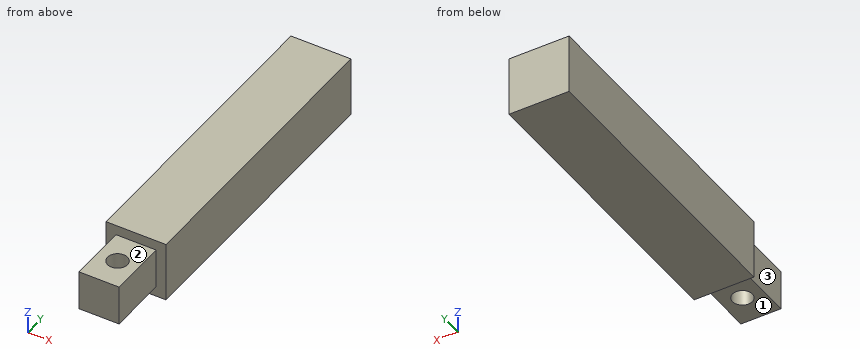
Autodesk Inventor part; units mm, degrees
ref_plane "YZ Plane" through (0, 0, 0) normal (1, 0, 0) x (0, 1, 0)
ref_plane "XZ Plane" through (0, 0, 0) normal (0, 1, 0) x (-1, 0, 0)
ref_plane "XY Plane" through (0, 0, 0) normal (0, 0, 1) x (1, 0, 0)
sketch "Sketch1" plane through (0, 0, 0) normal (0, 1, 0) x (-1, 0, 0)
  line L0 (0, 0) -> (-10, 0)
  line L1 (-10, 0) -> (-10, -10)
  line L2 (-10, -10) -> (0, -10)
  line L3 (0, -10) -> (0, 0)
  dimension "d0" = 10
  dimension "d1" = 10
extrude "Extrusion1" add sketch "Sketch1" along normal blind 15
sketch "Sketch2" plane through (0, 15, 0) normal (0, 1, 0) x (1, 0, 0)
  line L0 (12.5, -2.5) -> (-2.5, -2.5)
  line L1 (-2.5, -2.5) -> (-2.5, 12.5)
  line L2 (-2.5, 12.5) -> (12.5, 12.5)
  line L3 (12.5, 12.5) -> (12.5, -2.5)
  line L4 (12.5, -2.5) -> (-2.5, 12.5) construction
  line L5 (-2.5, -2.5) -> (12.5, 12.5) construction
  point P0 (0, 0)
  point P1 (5, 5)
  dimension "d4" = 15
  dimension "d5" = 15
extrude "Extrusion2" add sketch "Sketch2" along normal blind 75
sketch "Sketch3" plane through (0, 0, 0) normal (0, 0, 1) x (1, 0, 0)
  line L0 (0, 0) -> (0, 15)
  line L1 (0, 7.5) -> (10, 7.5)
  line L2 (10, 0) -> (10, 15)
  line L3 (-2.5, 15) -> (12.5, 15)
  line L4 (5, 15) -> (5, 0)
  line L5 (0, 0) -> (10, 0)
  point P0 (5, 7.5)
hole "Hole1" at (5, 7.5, 0) direction (0, 0, -1) diameter 5 end through all
properties part number "Pendulum"
Check sheet for the modelled part. Datum: model origin and axes. Units: mm. Face numbers are marked on the shaded views. A direction names the side the tool comes from. Round coordinates to 2 decimals unless told otherwise and drop trailing zeros. Write each loop counter-clockwise with the first axis right and the second up, starting at its lowest first coordinate (ties: lowest second). Pieces come first, ordered by that corner, then holes. Notation, with made-up numbers: (12, -26.75) -> (34, -26.75) arc R8 cw to (34, -20.75) -> close; hole circle Ø8 at (-1, 74). An arc over 180 degrees is marked (long way). Put each result on its own line as item: value.
(1) Sectioned sample at A-A (x = 5). Enter the section's corners in (y, z).
Values found:
outline: (0, -10) -> (5, -10) -> (5, 0) -> (0, 0) -> close; (10, -10) -> (15, -10) -> (15, -12.5) -> (90, -12.5) -> (90, 2.5) -> (15, 2.5) -> (15, 0) -> (10, 0) -> close
(2) Tool access check on the marked faces 1, 2 and 3. Record the directions out of +Z, -Z, +X, -X, +Y, -Y that give a thin tool (end or side, any length) a straight path to the whole face; none if there is none.
Values found:
face 1: -Z, +X, -X, -Y
face 2: +Z, +X, -X, -Y
face 3: +Z, -Z, -X, -Y
(3) Material ranges on line 1 (X direction, y = 7.5, z = -3.5); line 2 (Y direction, x = 5, z = -3.5); line 3 (Y direction, x = -1, z = 1), recorded low to high.
Values found:
line 1: x = 0 to 2.5, 7.5 to 10
line 2: y = 0 to 5, 10 to 90
line 3: y = 15 to 90
(4) Go/stop test with flat-tipped pins: pin 1 Ø8 at (x, y) = (5, 7.5) entering from +Z; pin 2 Ø3 at (y, z) = (6, -4.5) entering from -X; pin 3 Ø3 at (x, y) = (3.5, 6) entering from -Z. Record where each tip stops, or that it passes through.
Values found:
pin 1: stops at z = 0
pin 2: stops at x = 0
pin 3: stops at z = -10
(5) Sectioned sample at B-B (y = 7.5). Enter the section's corners in (x, z), plus the area to 3 significant figures.
Values found:
outline: (0, -10) -> (2.5, -10) -> (2.5, 0) -> (0, 0) -> close; (7.5, -10) -> (10, -10) -> (10, 0) -> (7.5, 0) -> close
area: 50.0 mm^2
